from build123d import *

# Parameters (mm, degrees)
SKETCH1_W                             = 106
SKETCH1_H                             = 95
BOSS_EXTRUDE1_DEPTH                   = 2
SKETCH4_W                             = 128.277926748
SKETCH4_H                             = 110.461548034
SKETCH4_W_2                           = 104
SKETCH4_H_2                           = 94
CUT_EXTRUDE1_DEPTH                    = 10
SKETCH6_W                             = 3.5
SKETCH6_H                             = 6.5
SKETCH6_W_2                           = 22.479668753
SKETCH6_H_2                           = 1.816385789
CUT_EXTRUDE2_DEPTH                    = 5
SKETCH8_R                             = 1.5
CUT_EXTRUDE3_DEPTH                    = 5
TAP_DRILL_FOR_M4X0_7_TAP2_D           = 3.3
TAP_DRILL_FOR_M4X0_7_TAP2_DEPTH       = 10
TAP_DRILL_FOR_M4X0_7_TAP2_CSINK_D     = 3.35
TAP_DRILL_FOR_M4X0_7_TAP2_CSINK_ANGLE = 90
TAP_DRILL_FOR_M4X0_7_TAP2_TIP         = 0.991420021


with BuildPart() as part:
    # Sketch1 → Boss-Extrude1 (new body)
    with BuildSketch(Plane.XY):
        Rectangle(SKETCH1_W, SKETCH1_H)
    extrude(amount=BOSS_EXTRUDE1_DEPTH)

    # Sketch4 → Cut-Extrude1 (cut)
    with BuildSketch(Plane(origin=(0, 0, 0), x_dir=(-1, 0, 0), z_dir=(0, 0, -1))):
        Rectangle(SKETCH4_W, SKETCH4_H)
        Rectangle(SKETCH4_W_2, SKETCH4_H_2, mode=Mode.SUBTRACT)
    extrude(amount=-CUT_EXTRUDE1_DEPTH, mode=Mode.SUBTRACT)

    # Sketch6 → Cut-Extrude2 (cut)
    with BuildSketch(Plane(origin=(0, 0, 0), x_dir=(-1, 0, 0), z_dir=(0, 0, -1))):
        with Locations((-50.25, -7.75)):
            Rectangle(SKETCH6_W, SKETCH6_H)
        with Locations((-50.25, 7.75)):
            Rectangle(SKETCH6_W, SKETCH6_H)
        with Locations((50.25, -7.75)):
            Rectangle(SKETCH6_W, SKETCH6_H)
        with Locations((50.25, 7.75)):
            Rectangle(SKETCH6_W, SKETCH6_H)
        with Locations((-41.239834377, -46.908192895)):
            Rectangle(SKETCH6_W_2, SKETCH6_H_2)
        with Locations((41.239834377, -46.908192895)):
            Rectangle(SKETCH6_W_2, SKETCH6_H_2)
        with Locations((-41.239834377, 46.908192895)):
            Rectangle(SKETCH6_W_2, SKETCH6_H_2)
        with Locations((41.239834377, 46.908192895)):
            Rectangle(SKETCH6_W_2, SKETCH6_H_2)
    extrude(amount=-CUT_EXTRUDE2_DEPTH, mode=Mode.SUBTRACT)

    # Sketch8 → Cut-Extrude3 (cut)
    with BuildSketch(Plane(origin=(0, 0, 0), x_dir=(-1, 0, 0), z_dir=(0, 0, -1))):
        with Locations((-45, 42)):
            Circle(SKETCH8_R)
        with Locations((-45, -24)):
            Circle(SKETCH8_R)
        with Locations((49, 42)):
            Circle(SKETCH8_R)
        with Locations((49, -24)):
            Circle(SKETCH8_R)
    extrude(amount=-CUT_EXTRUDE3_DEPTH, mode=Mode.SUBTRACT)

    # Tap Drill for M4x0.7 Tap2
    with Locations(Plane(origin=(0, 0, 0), x_dir=(-1, 0, 0), z_dir=(0, 0, -1))):
        with Locations((-15.008290978, 42.455982414), (-15.008290978, -42.455982414), (15.008290978, -42.455982414), (15.008290978, 42.455982414)):
            CounterSinkHole(TAP_DRILL_FOR_M4X0_7_TAP2_D / 2, TAP_DRILL_FOR_M4X0_7_TAP2_CSINK_D / 2, depth=TAP_DRILL_FOR_M4X0_7_TAP2_DEPTH, counter_sink_angle=TAP_DRILL_FOR_M4X0_7_TAP2_CSINK_ANGLE)
            with Locations((0, 0, -(TAP_DRILL_FOR_M4X0_7_TAP2_DEPTH + TAP_DRILL_FOR_M4X0_7_TAP2_TIP / 2))):  # 118° drill point
                Cone(0, TAP_DRILL_FOR_M4X0_7_TAP2_D / 2, TAP_DRILL_FOR_M4X0_7_TAP2_TIP, mode=Mode.SUBTRACT)


solid = part.part
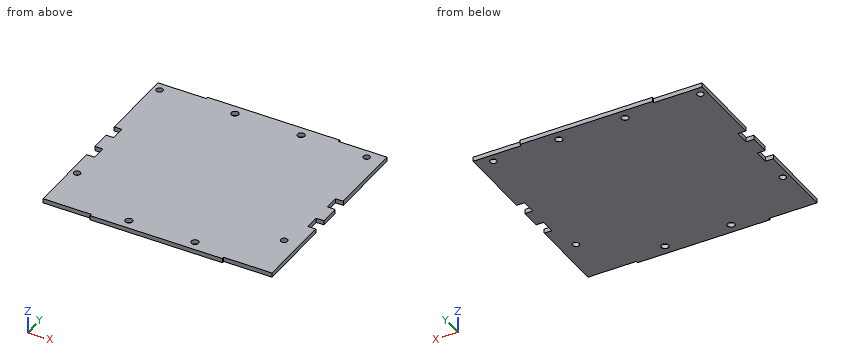
Design review of the part built by this model. Coordinates are the model's own, in mm. Round coordinates to 2 decimals unless told otherwise and drop trailing zeros. Write each loop counter-clockwise with the first axis right and the second up, starting at its lowest first coordinate (ties: lowest second). Pieces come first, ordered by that corner, then holes. Notation, with made-up numbers: (-21, 13.5) -> (38, 13.5) arc R13 ccw to (38, 31.5) -> close; hole circle Ø10 at (-23, 28). An arc over 180 degrees is marked (long way). One line per item, written item: value. Start each with the question number.
Q1. Add section D-D (z = 0.9). State how many separate pieces and enclosed holes the cut face has, then the cut area to 3 significant figures.
Q2. Add section A-A (y = -24). Give the boundary of the cut face in (x, z).
Q3. Add section C-C (x = 32). Give the boundary of the cut face in (y, z), then the cut area to 3 significant figures.
Q4. To check wall thickness, follow probe 1 along Y at (x, z) = (-49, 0.7); probe 2 along Y at (x, z) = (-31, 0.8); probe 3 along X at (y, z) = (-43, 1.4). State the ranges of each line that lie inside material, in increasing order.
Q5. Insertion check: P1, Ø1, axis at y = 6.5, z = 0.5, coming from the -X side; P2, Ø0.6, axis at x = -50, z = 1, coming from the -Y side; P3, Ø1, axis at x = 50.5, z = 1.5, coming from the +Y side. Each pin has a flat end and moves straight along its axis. Give the tip position at first contact, or say it passes through.
Q6. Add section B-B (x = 45). Give the boundary of the cut face in (y, z).
Response:
1. separate pieces: 1
1. enclosed holes: 8
1. area: 9,530 mm^2
2. outline: (-52, 0) -> (-50.5, 0) -> (-50.5, 2) -> (-52, 2) -> close; (-47.5, 0) -> (43.5, 0) -> (43.5, 2) -> (-47.5, 2) -> close; (46.5, 0) -> (52, 0) -> (52, 2) -> (46.5, 2) -> close
3. outline: (-46, 0) -> (46, 0) -> (46, 2) -> (-46, 2) -> close
3. area: 184 mm^2
4. probe 1: y = -46 to -25.5, -22.5 to -11, -4.5 to 4.5, 11 to 40.5, 43.5 to 46
4. probe 2: y = -46 to 46
4. probe 3: x = -52 to -16.57, -13.45 to 13.45, 16.57 to 52
5. P1: stops at x = -48.5
5. P2: stops at y = -46
5. P3: stops at y = 46
6. outline: (-46, 0) -> (-25.5, 0) -> (-25.5, 2) -> (-46, 2) -> close; (-22.5, 0) -> (40.5, 0) -> (40.5, 2) -> (-22.5, 2) -> close; (43.5, 0) -> (46, 0) -> (46, 2) -> (43.5, 2) -> close
